Model file for the job. Use its own axes, mm. A direction names the side the tool comes from. Round coordinates to 2 decimals unless told otherwise and drop trailing zeros. Order: outer loops, then holes, each group sorted by start corner. A loop starts at its lowest first (then second) coordinate and runs counter-clockwise, first axis right, second up. Notation, with made-up numbers: M 62.5,54.5 L 71.5,54.5 A21 cw 71.5,65.5 Z; hole C -14,-38 d5. An arc over 180 degrees is marked long. Return JSON: item names as keys, results as strings. Group by question number.
Item 1: Pin check, flat tips, straight feed: pin 1 Ø1.5 at (y, z) = (24, -56.5) entering from +X; pin 2 Ø2 at (x, z) = (14, -80.5) entering from +Y. Stop position of each tip, or through.
Item 2: Probe line 1 along Z through (x, y) = (13, 23) (3 decimals); line 2 along X through (y, z) = (25, -74); line 3 along Y through (x, z) = (15.5, -59). List the from-to ranges inside material, lowest first.
Item 3: Slice it at C-C on z = -53. Write the cut outline in (x, y) (3 decimals), then the cut area to 3 significant figures.
Item 4: Pull direction Z, two halves, no side cores. Call faces 4 (the face through (15, 27, 3.175)), 5 (the face through (15.685, 21.807, -87.046)), 6 (the face through (15, 25, -93.446)): pulls with the +Z half, pulls with the -Z half, needs draft (parallel to the pull), parting line crosses it, or undercut.
Item 5: Slice it at A-A on y = 25.75. Write the cut outline in (x, z) (3 decimals).
Item 6: Which spindle directions (+Z, -Z, +X, -X, +Y, -Y) get a long thin tool onto all of the face, cutting with end or side? Do faces 1 (the face through (14.358, 26.522, 8.584)), 2 (the face through (15, 25, 13.843)), 3 (the face through (15.685, 21.807, -14.333)). Say none if no direction does.
Item 7: Slice it at B-B on x = 16. Write the cut outline in (y, z) (3 decimals).
from build123d import *


with BuildPart() as part:
    # Sketch1 → Revolve1 (revolve)
    with BuildSketch(Plane(origin=(15.304322218, 0, 0), x_dir=(0, 0, -1), z_dir=(1, 0, 0)), mode=Mode.PRIVATE) as revolve1_sk:
        Polygon((13.97, 27.878467802), (-3.175, 27.878467802), (-3.175, 26.753467802), (-13.843, 26.753467802), (-13.843, 24.703467802), (93.445553682, 24.703467802), (93.445553682, 27.878467802), (87.419403682, 27.878467802), (87.419403682, 27.624467802), (86.682803682, 27.624467802), (86.682803682, 27.878467802), (65.655613748, 27.878467802), (14.7066, 27.878467802), (14.7066, 27.624467802), (13.97, 27.624467802), align=None)
    revolve(revolve1_sk.sketch.rotate(Axis((15.304322218, 24.703467802, -93.445553682), (0, 0, 1)), 90), axis=Axis((15.304322218, 24.703467802, -93.445553682), (0, 0, 1)))


solid = part.part
Output values:
{
 "1": {"pin 1": "x = 18.48", "pin 2": "y = 27.86"},
 "2": {"line 1": "-93.446 to 3.175", "line 2": "12.14 to 18.47", "line 3": "21.53 to 27.87"},
 "3": {"outline": "C 15.304,24.703 d6.35", "area": "31.7 mm²"},
 "4": {"face 4": "pulls with the +Z half", "face 5": "undercut", "face 6": "pulls with the -Z half"},
 "5": {"outline": "M 12.307,-93.446 L 18.302,-93.446 L 18.302,-87.419 L 18.031,-87.419 L 18.031,-86.683 L 18.302,-86.683 L 18.302,-14.707 L 18.031,-14.707 L 18.031,-13.97 L 18.302,-13.97 L 18.302,3.175 L 17.067,3.175 L 17.067,13.843 L 13.542,13.843 L 13.542,3.175 L 12.307,3.175 L 12.307,-13.97 L 12.577,-13.97 L 12.577,-14.707 L 12.307,-14.707 L 12.307,-86.683 L 12.577,-86.683 L 12.577,-87.419 L 12.307,-87.419 Z"},
 "6": {"face 1": "+Z", "face 2": "+Z, +X, -X, +Y, -Y", "face 3": "none"},
 "7": {"outline": "M 21.606,-93.446 L 27.801,-93.446 L 27.801,-87.419 L 27.54,-87.419 L 27.54,-86.683 L 27.801,-86.683 L 27.801,-14.707 L 27.54,-14.707 L 27.54,-13.97 L 27.801,-13.97 L 27.801,3.175 L 26.632,3.175 L 26.632,13.843 L 22.775,13.843 L 22.775,3.175 L 21.606,3.175 L 21.606,-13.97 L 21.867,-13.97 L 21.867,-14.707 L 21.606,-14.707 L 21.606,-86.683 L 21.867,-86.683 L 21.867,-87.419 L 21.606,-87.419 Z"}
}
